The figure shows three views and two pictorial views of one solid part (mm, origin at its lowest corner). Answer the questions. A direction names the side the tool comes from. Give positions to 0.01 mm unless a question says otherwise; leave off trailing zeros. Loops run counter-clockwise (first coordinate to the right, second up) from the corner with the lowest first, then second, coordinate; pieces in that order, holes last. Notation, with made-up numbers: M -9.75,-35 L 36.25,-35 A20 ccw 36.25,-28 Z; hole C 46,21 d9. An arc over 180 degrees is marked long. One line per item, written item: value. Start each with the question number.
Q1. A cutting plane is placed at B-B, the plane x = 12. Determine the outline of the cut face in (y, z), and give its area (3 significant figures).
Q2. A cutting plane is placed at C-C, the plane y = 78.5. Determine the outline of the cut face in (x, z).
Q3. The mould has two halves that part along Y. Classify the marked faces 1, 2 and 3: +Y half, -Y half, draft (parallel to the pull), parting line (faces both ways), or undercut.
Q4. For the marked faces 4 and 5, determine the directions among +Z, -Z, +X, -X, +Y, -Y from which every point of the face is accessible in a straight line to the end or side of a thin tool.
Q5. Consider L1, parallel to X at y = 48.5, z = 1; L2, parallel to Y at x = 20.5, z = 1.3; L3, parallel to X at y = 48, z = 1. Determine where each line is inside the solid, lowest interval first.
Q6. Flat-ended cylindrical pins translate along their axes: pin 1 (9 mm diameter, centred on x = 4.5, y = 52, fed in from +Z); pin 2 (1.5 mm diameter, centred on x = 20.5, y = 49, fed in from -Z); pin 3 (9.5 mm diameter, centred on y = 68, z = 29, fed in from -X). Find the tip coordinate at first contact, or state that the pin passes through.
Q7. A cutting plane is placed at A-A, the plane z = 26. Determine the outline of the cut face in (x, y), and give its area (3 significant figures).
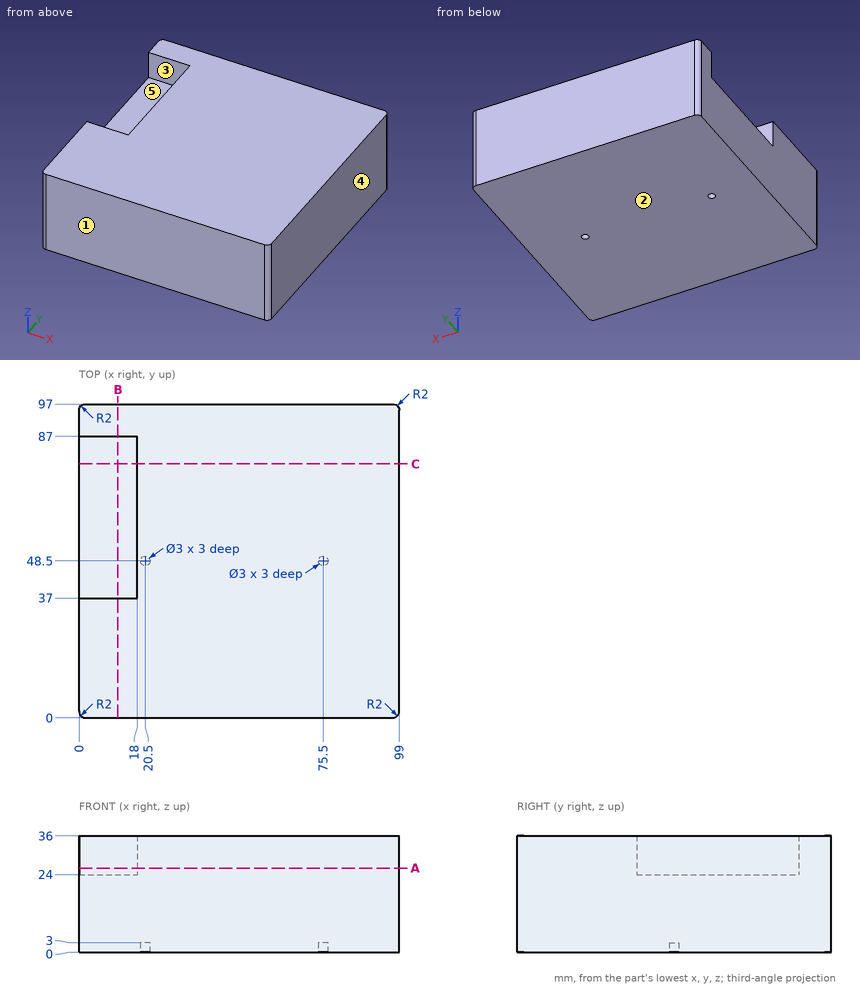
Answer block:
1. outline: M 0,0 L 97,0 L 97,36 L 87,36 L 87,24 L 37,24 L 37,36 L 0,36 Z
1. area: 2,890 mm^2
2. outline: M 0,0 L 99,0 L 99,36 L 18,36 L 18,24 L 0,24 Z
3. face 1: -Y half
3. face 2: draft
3. face 3: undercut
4. face 4: +Z, -Z, +X, +Y, -Y
4. face 5: +Z, -X
5. L1: 0 to 19, 22 to 74, 77 to 99
5. L2: 0 to 47, 50 to 97
5. L3: 0 to 19.09, 21.91 to 74.09, 76.91 to 99
6. pin 1: z = 24
6. pin 2: z = 3
6. pin 3: x = 18
7. outline: M 0,2 A2 ccw 2,0 L 97,0 A2 ccw 99,2 L 99,95 A2 ccw 97,97 L 2,97 A2 ccw 0,95 L 0,87 L 18,87 L 18,37 L 0,37 Z
7. area: 8,700 mm^2
